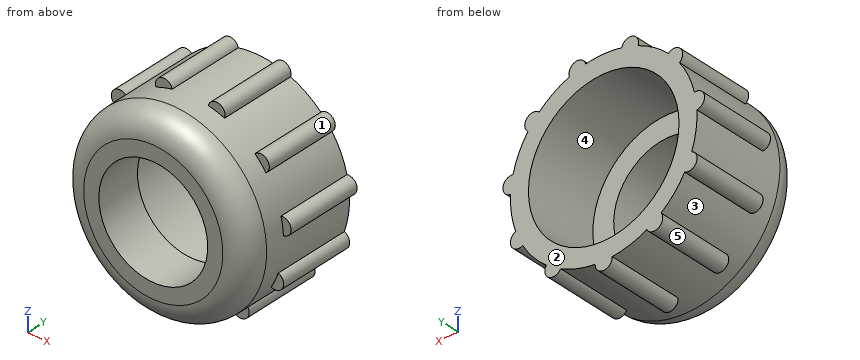
```python
from build123d import *

# Parameters (mm, degrees)
SKETCH1_R           = 25.019
BOSS_EXTRUDE1_DEPTH = 32.512
SKETCH2_R           = 14.605
CUT_EXTRUDE1_DEPTH  = 32.512
BOSS_EXTRUDE2_START = -20.828
BOSS_EXTRUDE2_DEPTH = 20.828
CIRPATTERN1_COUNT   = 11
FILLET1_R           = 6.35
SKETCH4_R           = 20.193
CUT_EXTRUDE2_DEPTH  = 20.32


with BuildPart() as part:
    # Sketch1 → Boss-Extrude1 (new body)
    with BuildSketch(Plane(origin=(0, 0, 0), x_dir=(1, 0, 0), z_dir=(0, 1, 0))):
        with Locations(Location((0, 0, 0), (0, 0, 270))):
            Circle(SKETCH1_R)
    extrude(amount=BOSS_EXTRUDE1_DEPTH)

    # Sketch2 → Cut-Extrude1 (cut)
    with BuildSketch(Plane(origin=(0, 32.512, 0), x_dir=(1, 0, 0), z_dir=(0, 1, 0))):
        with Locations(Location((0, 0, 0), (0, 0, 270))):
            Circle(SKETCH2_R)
    extrude(amount=-CUT_EXTRUDE1_DEPTH, mode=Mode.SUBTRACT)

    # Sketch3 → Boss-Extrude2 (add)
    with BuildSketch(Plane(origin=(0, 32.512, 0), x_dir=(1, 0, 0), z_dir=(0, 1, 0)).offset(BOSS_EXTRUDE2_START)):
        with BuildLine():
            ThreePointArc((2.283613147, 24.914563452), (0, 25.019), (-2.283613147, 24.914563452))
            ThreePointArc((-2.283613147, 24.914563452), (0, 27.305), (2.283613147, 24.914563452))
        make_face()
    boss_extrude2 = extrude(amount=BOSS_EXTRUDE2_DEPTH)

    # CirPattern1: Boss-Extrude2 ×11 about axis
    cirpattern1_axis = Axis((0, 0, 0), (0, 1, 0))
    for i in range(1, CIRPATTERN1_COUNT):
        add(boss_extrude2.rotate(cirpattern1_axis, i * 360 / CIRPATTERN1_COUNT))

    # Fillet1
    fillet1_edges = [part.edges().sort_by_distance(p)[0] for p in [
        (0, 0, -25.019),
    ]]
    fillet(fillet1_edges, radius=FILLET1_R)

    # Sketch4 → Cut-Extrude2 (cut)
    with BuildSketch(Plane(origin=(0, 32.512, 0), x_dir=(1, 0, 0), z_dir=(0, 1, 0))):
        with Locations(Location((0, 0, 0), (0, 0, 270))):
            Circle(SKETCH4_R)
    extrude(amount=-CUT_EXTRUDE2_DEPTH, mode=Mode.SUBTRACT)


solid = part.part
```
Verification items for the finished model (mm, model axes). Face numbers are marked on the shaded views. A direction names the side the tool comes from. Coordinates: 2 decimals unless noted, no trailing zeros. Order: outer loops, then holes, each group sorted by start corner. A loop starts at its lowest first (then second) coordinate and runs counter-clockwise, first axis right, second up. Notation, with made-up numbers: (5, -12.75) -> (9, -12.75) arc R18 ccw to (9, -5.75) -> close; hole circle Ø10 at (56, -20). An arc over 180 degrees is marked (long way). Answer as CSV lines item,"result". Start each with the question number.
1) Gauge pin test, flat ends, axial feed: pin 1 Ø3 at (x, z) = (-10, 15.5) entering from -Y; pin 2 Ø5 at (x, y) = (-3.5, 10.5) entering from -Z; pin 3 Ø5 at (y, z) = (9, 4.5) entering from +X; pin 4 Ø1.2 at (x, z) = (1, -26.5) entering from -Y. Record the tip position at first contact, or that the pin passes through.
2) Cross-section at B-B, the plane z = 0. Record the boundary of the cut face in (x, y) (3 decimals).
3) Material ranges on L1, parallel to X at y = 21.25, z = 0; L2, parallel to X at y = 9.5, z = 7; L3, parallel to Z at x = -11, y = 30.5, recorded low to high. Write a range as [from, to].
4) Set-up check for the marked faces 4 and 5: record each of +Z, -Z, +X, -X, +Y, -Y from which the full face is reachable in a straight line by a thin tool's end or side.
5) Cross-section at A-A, the plane x = 0. Record the boundary of the cut face in (y, z) (3 decimals).
6) Release check for a two-part mould opening along Z. For the marked faces 1, 2 and 3 record: released by +Z, released by -Z, zero draft, split by the parting line, or undercut.
7) Cross-section at C-C, the plane y = 30.5. Record the boundary of the cut face in (x, z).
8) Cross-section at D-D, the plane y = 3.5. Record the boundary of the cut face in (x, z) (1 decimal), then the cut area to 3 significant figures.
Conclusion:
1,pin 1,"stops at y = 0"
1,pin 2,"stops at z = -26.9"
1,pin 3,"stops at x = 24.94"
1,pin 4,"stops at y = 11.68"
2,outline,"(-25.019, 6.35) arc R6.35 ccw to (-18.669, 0) -> (-14.605, 0) -> (-14.605, 12.192) -> (-20.193, 12.192) -> (-20.193, 32.512) -> (-25.019, 32.512) -> close; (14.605, 0) -> (18.669, 0) arc R6.35 ccw to (25.019, 6.35) -> (25.019, 32.512) -> (20.193, 32.512) -> (20.193, 12.192) -> (14.605, 12.192) -> close"
3,L1,"x = [-25.02, -20.19], [20.19, 25.02]"
3,L2,"x = [-24.02, -12.82], [12.82, 24.02]"
3,L3,"z = [-22.47, -16.93], [16.93, 22.47]"
4,face 4,"+Y"
4,face 5,"+Y, -Y"
5,outline,"(0, -18.669) arc R6.35 ccw to (6.35, -25.019) -> (11.684, -25.019) -> (11.684, -27.305) -> (32.512, -27.305) -> (32.512, -20.193) -> (12.192, -20.193) -> (12.192, -14.605) -> (0, -14.605) -> close; (0, 14.605) -> (12.192, 14.605) -> (12.192, 20.193) -> (32.512, 20.193) -> (32.512, 25.019) -> (6.35, 25.019) arc R6.35 ccw to (0, 18.669) -> close"
6,face 1,"undercut"
6,face 2,"zero draft"
6,face 3,"undercut"
7,outline,"(-24.99, 1.29) arc R25.02 ccw to (-23.61, -8.27) arc R2.29 ccw (long way) to (-21.71, -12.43) arc R25.02 ccw to (-15.39, -19.72) arc R2.29 ccw (long way) to (-11.55, -22.19) arc R25.02 ccw to (-2.28, -24.91) arc R2.29 ccw (long way) to (2.28, -24.91) arc R25.02 ccw to (11.55, -22.19) arc R2.29 ccw (long way) to (15.39, -19.72) arc R25.02 ccw to (21.71, -12.43) arc R2.29 ccw (long way) to (23.61, -8.27) arc R25.02 ccw to (24.99, 1.29) arc R2.29 ccw (long way) to (24.34, 5.81) arc R25.02 ccw to (20.32, 14.59) arc R2.29 ccw (long way) to (17.33, 18.04) arc R25.02 ccw to (9.21, 23.26) arc R2.29 ccw (long way) to (4.83, 24.55) arc R25.02 ccw to (-4.83, 24.55) arc R2.29 ccw (long way) to (-9.21, 23.26) arc R25.02 ccw to (-17.33, 18.04) arc R2.29 ccw (long way) to (-20.32, 14.59) arc R25.02 ccw to (-24.34, 5.81) arc R2.29 ccw (long way) to start; hole circle Ø40.39 at (0, 0)"
8,outline,"circle Ø48.7 at (0, 0); hole circle Ø29.2 at (0, 0)"
8,area,"1,190 mm²"
